Work out the finished part from the listing and answer in its coordinate system (mm). Give positions to 0.01 mm unless a question says otherwise; leave off trailing zeros. Loops run counter-clockwise (first coordinate to the right, second up) from the corner with the lowest first, then second, coordinate; pieces in that order, holes last. Notation, with made-up numbers: M 83.5,9 L 91.5,9 A29 ccw 91.5,46 Z; hole C 30.5,-35.75 d3. An arc over 180 degrees is marked long. Use a Markdown table: item, result.
Autodesk Inventor part; units mm, degrees
ref_plane "YZ Plane" through (0, 0, 0) normal (1, 0, 0) x (0, 1, 0)
ref_plane "XZ Plane" through (0, 0, 0) normal (0, 1, 0) x (-1, 0, 0)
ref_plane "XY Plane" through (0, 0, 0) normal (0, 0, 1) x (1, 0, 0)
sketch "スケッチ1" plane through (0, 0, 0) normal (0, 1, 0) x (-1, 0, 0)
  line L0 (0, 0) -> (-15, 0)
  line L1 (-15, 0) -> (-15, 0.5)
  line L2 (-15, 0.5) -> (0, 0.5)
  line L3 (0, 0.5) -> (0, 0)
  circle A0 centre (0, -5) radius 5
  circle A1 centre (0, -5) radius 5.5
  line L4 (1.2941, -9.8296) -> (-32.5133, -18.8883)
  line L5 (-32.5133, -18.8883) -> (-32.3839, -19.3713)
  line L6 (-32.3839, -19.3713) -> (1.4235, -10.3126)
  point P0 (-0.2935, -9.9914)
  point P1 (-0.9191, -10.4227)
  point P2 (-2.2913, 0)
  dimension "d3" = 10
  dimension "d2" = 11
  dimension "d4" = 15
  dimension "d5" = 35
  dimension "d6" = 15
extrude "押し出し1" add sketch "スケッチ1" along normal blind 5 contours L0 A1 L3 | L3 A1 L4 A0 | L0 L1 L2 A1 | A1 L6 L5 L4
properties part number "bend_sensor"
(1) A cutting plane is placed at C-C (z = -8). Write down the section's boundary in (x, y).
Entries:
| item | result |
|---|---|
| outline | M -4.61,0 L -4,0 L -4,5 L -4.61,5 Z |
(2) Given P1, Ø0.7, axis at x = 0.5, y = 2, coming from the -Z side; P2, Ø2, axis at y = 1.5, z = -8.5, coming from the -X side; P3, Ø0.6, axis at y = 2.5, z = 0, coming from the +X side, each flat-ended and moving along its own axis, determine where each tip first touches the part or whether it passes through.
Entries:
| item | result |
|---|---|
| P1 | stops at z = -10.92 |
| P2 | stops at x = -4.9 |
| P3 | stops at x = 15 |
(3) A cutting plane is placed at A-A (x = 8). Write down the section's boundary in (y, z), and give its area (3 significant figures).
Entries:
| item | result |
|---|---|
| outline | M 0,-12.84 L 5,-12.84 L 5,-12.32 L 0,-12.32 Z; M 0,0 L 5,0 L 5,0.5 L 0,0.5 Z |
| area | 5.09 mm² |
(4) A cutting plane is placed at B-B (y = 3.95). Write down the section's boundary in (x, z).
Entries:
| item | result |
|---|---|
| outline | M -1.42,-10.31 L 32.38,-19.37 L 32.51,-18.89 L -1.29,-9.83 A5 cw 0,0 L 15,0 L 15,0.5 L 0,0.5 A5.5 ccw Z |
(5) Consider probe 1 along Z at (x, y) = (-2, 3.9); probe 2 along Z at (x, y) = (9, 4.2); probe 3 along Z at (x, y) = (19, 1.85). Determine where each line is inside the solid, lowest interval first. Write a range as [from, to].
Entries:
| item | result |
|---|---|
| probe 1 | z = [-10.12, -9.58], [-0.42, 0.12] |
| probe 2 | z = [-13.11, -12.59], [0, 0.5] |
| probe 3 | z = [-15.79, -15.27] |
(6) A cutting plane is placed at D-D (x = 22.5). Write down the section's boundary in (y, z), and give its area (3 significant figures).
Entries:
| item | result |
|---|---|
| outline | M 0,-16.72 L 5,-16.72 L 5,-16.21 L 0,-16.21 Z |
| area | 2.59 mm² |
